from build123d import *

# Parameters (mm, degrees)
SKETCH1_W           = 70
SKETCH1_H           = 70
BOSS_EXTRUDE1_DEPTH = 2
SKETCH2_W           = 2
SKETCH2_H           = 20
BOSS_EXTRUDE2_DEPTH = 2
SKETCH3_W           = 20
SKETCH3_H           = 2
CUT_EXTRUDE1_DEPTH  = 2
SKETCH4_W           = 12.9
SKETCH4_H           = 7
CUT_EXTRUDE2_DEPTH  = 10


with BuildPart() as part:
    # Sketch1 → Boss-Extrude1 (new body)
    with BuildSketch(Plane.XY):
        Rectangle(SKETCH1_W, SKETCH1_H)
    extrude(amount=-BOSS_EXTRUDE1_DEPTH)

    # Sketch2 → Boss-Extrude2 (add)
    with BuildSketch(Plane.XY):
        with Locations((-36, 15)):
            Rectangle(SKETCH2_W, SKETCH2_H)
        with Locations((-36, -15)):
            Rectangle(SKETCH2_W, SKETCH2_H)
        with Locations((36, -15)):
            Rectangle(SKETCH2_W, SKETCH2_H)
        with Locations((36, 15)):
            Rectangle(SKETCH2_W, SKETCH2_H)
    extrude(amount=-BOSS_EXTRUDE2_DEPTH)

    # Sketch3 → Cut-Extrude1 (cut)
    with BuildSketch(Plane.XY):
        with Locations((-15, 34)):
            Rectangle(SKETCH3_W, SKETCH3_H)
        with Locations((15, 34)):
            Rectangle(SKETCH3_W, SKETCH3_H)
        with Locations((-15, -34)):
            Rectangle(SKETCH3_W, SKETCH3_H)
        with Locations((15, -34)):
            Rectangle(SKETCH3_W, SKETCH3_H)
    extrude(amount=-CUT_EXTRUDE1_DEPTH, mode=Mode.SUBTRACT)

    # Sketch4 → Cut-Extrude2 (cut)
    with BuildSketch(Plane.XY):
        Rectangle(SKETCH4_W, SKETCH4_H)
    extrude(amount=-CUT_EXTRUDE2_DEPTH, mode=Mode.SUBTRACT)


solid = part.part
Read the model definition and answer for the solid it produces. Units are mm, in the model's axes. A direction names the side the tool comes from. Coordinates: 2 decimals unless noted, no trailing zeros. Order: outer loops, then holes, each group sorted by start corner. A loop starts at its lowest first (then second) coordinate and runs counter-clockwise, first axis right, second up. Notation, with made-up numbers: M 46,-38.5 L 105,-38.5 A12 ccw 105,-20.5 Z; hole C -1.75,-35.75 d2. An arc over 180 degrees is marked long. Put each result on its own line as item: value. Start each with the question number.
Item 1: Given pin 1 Ø1 at (y, z) = (-34.5, -1) entering from +X; pin 2 Ø0.6 at (y, z) = (-1.5, -1.5) entering from -X; pin 3 Ø1 at (x, z) = (18.5, -0.5) entering from +Y, each flat-ended and moving along its own axis, determine where each tip first touches the part or whether it passes through.
Item 2: The mould has two halves that part along X. Classify faces 1 (the face through (0, -3.5, -1)), 2 (the face through (30, -35, -1)), 3 (the face through (37, -15, -1)), 4 (the face through (-25, -34, -1)): +X half, -X half, draft (parallel to the pull), parting line (faces both ways), or undercut.
Item 3: Section D-D, the plane y = -28.5 is taken. Determine the outline of the cut face in (x, z).
Item 4: Consider probe 1 along Y at (x, z) = (1.5, -1.25); probe 2 along Y at (x, z) = (6, -1.1); probe 3 along Y at (x, z) = (-18, -1.55). Determine where each line is inside the solid, lowest interval first. Write a range as [from, to].
Item 5: Section C-C, the plane x = 20 is taken. Determine the outline of the cut face in (y, z), plus the area to 3 significant figures.
Item 6: Section B-B, the plane y = 1 is taken. Determine the outline of the cut face in (x, z), plus the area to 3 significant figures.
Item 7: For faces 5 (the face through (-15, -33, -1)), 6 (the face through (-36, 5, -1)), 7 (the face through (-25, 34, -1)), 8 (the face through (35, 30, -1)), 9 (the face through (35, -30, -1)), determine the directions among +Z, -Z, +X, -X, +Y, -Y from which every point of the face is accessible in a straight line to the end or side of a thin tool.
Item 8: Section A-A, the plane x = -0.5 is taken. Determine the outline of the cut face in (y, z), plus the area to 3 significant figures.
Computed:
1. pin 1: stops at x = 35
1. pin 2: stops at x = -35
1. pin 3: stops at y = 33
2. face 1: undercut
2. face 2: draft
2. face 3: +X half
2. face 4: undercut
3. outline: M -35,-2 L 35,-2 L 35,0 L -35,0 Z
4. probe 1: y = [-35, -3.5], [3.5, 35]
4. probe 2: y = [-33, -3.5], [3.5, 33]
4. probe 3: y = [-33, 33]
5. outline: M -33,-2 L 33,-2 L 33,0 L -33,0 Z
5. area: 132 mm2
6. outline: M -35,-2 L -6.45,-2 L -6.45,0 L -35,0 Z; M 6.45,-2 L 35,-2 L 35,0 L 6.45,0 Z
6. area: 114 mm2
7. face 5: +Z, -Z, -Y
7. face 6: +Z, -Z, -X
7. face 7: +Z, -Z, +Y
7. face 8: +Z, -Z, +X, +Y
7. face 9: +Z, -Z, +X, -Y
8. outline: M -35,-2 L -3.5,-2 L -3.5,0 L -35,0 Z; M 3.5,-2 L 35,-2 L 35,0 L 3.5,0 Z
8. area: 126 mm2
